```python
from build123d import *

# Parameters (mm, degrees)
SKETCH2_W           = 102
SKETCH2_H           = 42.5
BOSS_EXTRUDE1_DEPTH = 5
SKETCH3_W           = 97.3
SKETCH3_H           = 38.1
CUT_EXTRUDE1_DEPTH  = 3.5
SKETCH4_W           = 2.8
SKETCH4_H           = 6.8
BOSS_EXTRUDE3_DEPTH = 2.3
CUT_EXTRUDE4_DEPTH  = 2
SKETCH9_R           = 0.85
CUT_EXTRUDE5_DEPTH  = 31
FILLET1_R           = 2


with BuildPart() as part:
    # Sketch2 → Boss-Extrude1 (new body)
    with BuildSketch(Plane.XY):
        with Locations((51, 21.25)):
            Rectangle(SKETCH2_W, SKETCH2_H)
    extrude(amount=BOSS_EXTRUDE1_DEPTH)

    # Sketch3 → Cut-Extrude1 (cut)
    with BuildSketch(Plane.XY.offset(5)):
        with Locations((51.45, 21.25)):
            Rectangle(SKETCH3_W, SKETCH3_H)
    extrude(amount=-CUT_EXTRUDE1_DEPTH, mode=Mode.SUBTRACT)

    # Sketch4 → Boss-Extrude3 (add)
    with BuildSketch(Plane.XY.offset(5)):
        with Locations((1.4, 28.4635072)):
            Rectangle(SKETCH4_W, SKETCH4_H)
    extrude(amount=BOSS_EXTRUDE3_DEPTH)

    # Sketch8 → Cut-Extrude4 (cut)
    with BuildSketch(Plane.XY.offset(5)):
        Polygon((2.8, 31.8635072), (1.8, 31.8635072), (1.8, 41.3), (101.1, 41.3), (101.1, 1.2), (1.8, 1.2), (1.8, 25.0635072), (2.8, 25.0635072), (2.8, 2.2), (100.1, 2.2), (100.1, 40.3), (2.8, 40.3), align=None)
    extrude(amount=-CUT_EXTRUDE4_DEPTH, mode=Mode.SUBTRACT)

    # Sketch9 → Cut-Extrude5 (cut)
    with BuildSketch(Plane.XY.offset(1.5)):
        with Locations((12, 21.25)):
            Circle(SKETCH9_R)
    extrude(amount=-CUT_EXTRUDE5_DEPTH, mode=Mode.SUBTRACT)

    # Fillet1
    fillet1_edges = [part.edges().sort_by_distance(p)[0] for p in [
        (51, 42.5, 0),
        (51, 0, 0),
    ]]
    fillet(fillet1_edges, radius=FILLET1_R)


solid = part.part
```
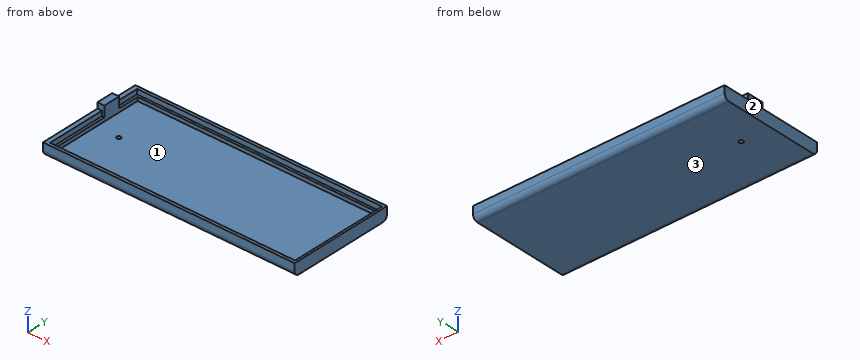
The model under review builds one solid part; all positions refer to its coordinate system, in mm. Face numbers are marked on the shaded views. Give positions to 0.01 mm unless a question says otherwise; leave off trailing zeros. Order: outer loops, then holes, each group sorted by start corner. A loop starts at its lowest first (then second) coordinate and runs counter-clockwise, first axis right, second up. Notation, with made-up numbers: (-9.75, 60.25) - (32.25, 60.25) arc R5 ccw to (32.25, 66.25) - close; hole circle Ø11 at (45, -32.5). An arc over 180 degrees is marked (long way). Use CSV: the item, a comma, the result in double quotes. Start each with the question number.
Q1. We need section C-C, the plane z = 6.25. Write out the cut boundary in (x, y).
Q2. We need section B-B, the plane x = 28. Write out the cut boundary in (y, z), and give its area (3 significant figures).
Q3. To check wall thickness, follow line 1 along X through (y, z) = (8, 3.25); line 2 along X through (y, z) = (13, 2); line 3 along Z through (x, y) = (42.5, 21). State the ranges of each line that lie inside material, in increasing order. Write a range as [from, to].
Q4. The part is to be moulded in two halves that separate along X. For the marked faces 1, 2 and 3, say which applies: +X half, -X half, draft (parallel to the pull), parting line (faces both ways), or undercut.
Q5. Clearance check with a flat-ended pin moving along its axis: pin 1 Ø1.5 at (x, y) = (66.5, 23) entering from +Z. State where the tip first meets the part, or that it passes through.
Q6. We need section A-A, the plane y = 13.5. Write out the cut boundary in (x, z).
Outcome:
1,outline,"(0, 25.06) - (2.8, 25.06) - (2.8, 31.86) - (0, 31.86) - close"
2,outline,"(0, 2) arc R2 ccw to (2, 0) - (40.5, 0) arc R2 ccw to (42.5, 2) - (42.5, 5) - (41.3, 5) - (41.3, 3) - (40.3, 3) - (40.3, 1.5) - (2.2, 1.5) - (2.2, 3) - (1.2, 3) - (1.2, 5) - (0, 5) - close"
2,area,"73.4 mm^2"
3,line 1,"x = [0, 1.8], [101.1, 102]"
3,line 2,"x = [0, 2.8], [100.1, 102]"
3,line 3,"z = [0, 1.5]"
4,face 1,"undercut"
4,face 2,"-X half"
4,face 3,"draft"
5,pin 1,"stops at z = 1.5"
6,outline,"(0, 0) - (102, 0) - (102, 5) - (101.1, 5) - (101.1, 3) - (100.1, 3) - (100.1, 1.5) - (2.8, 1.5) - (2.8, 3) - (1.8, 3) - (1.8, 5) - (0, 5) - close"
